from build123d import *

# Parameters (mm, degrees)
F0_R     = 2.013664
F1_DEPTH = 0.508
F2_R     = 2.54


with BuildPart() as f1:
    # F0 (on Top) → F1 (new body)
    with BuildSketch(Plane.XY):
        Polygon((5.08, 9.940335), (-3.64114, 9.940335), (-4.115906, 9.940335), (-4.115906, -0.219665), (5.08, -0.219665), align=None)
        with Locations((0, 5.06829)):
            Circle(F0_R, mode=Mode.SUBTRACT)
    extrude(amount=F1_DEPTH)

    # F2
    f2_edges = [f1.edges().sort_by_distance(p)[0] for p in [
        (5.08, 9.940335, 0.254),
        (5.08, -0.219665, 0.254),
    ]]
    fillet(f2_edges, radius=F2_R)


solid = f1.part
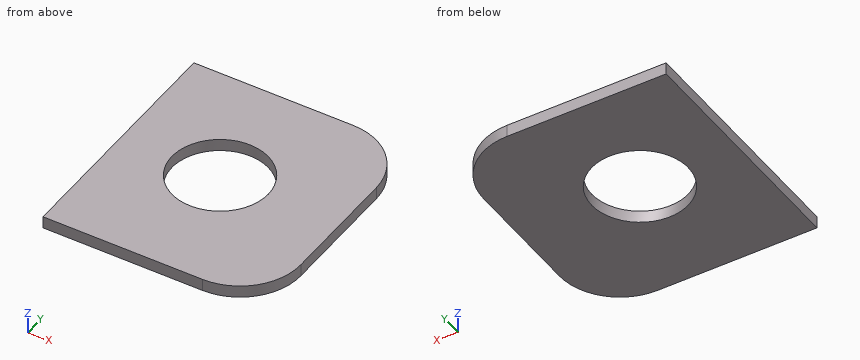
Design review of the part built by this model. Coordinates are the model's own, in mm. Round coordinates to 2 decimals unless told otherwise and drop trailing zeros. Write each loop counter-clockwise with the first axis right and the second up, starting at its lowest first coordinate (ties: lowest second). Pieces come first, ordered by that corner, then holes. Notation, with made-up numbers: (49.25, 43) - (92.25, 43) arc R19 cw to (92.25, 67) - close; hole circle Ø2 at (16.5, 88.25). An arc over 180 degrees is marked (long way). Use a Markdown table: item, result. Add a question column.
1. We need section D-D (y = 9.5). State the section outline as (x, z) points.
2. We need section A-A (x = 0). State the section outline as (y, z) points, then the cut area to 3 significant figures.
3. Wall thickness on probe 1 along Y at (x, z) = (0, 0.35); probe 2 along X at (y, z) = (5, 0.1); probe 3 along X at (y, z) = (3.75, 0.2): over which ranges is each line inside the solid? List them lowest first.
4. We need section C-C (z = 0.2). State the section outline as (x, y) points, then the cut area to 3 significant figures.
5. We need section B-B (y = 4.25). State the section outline as (x, z) points, then the cut area to 3 significant figures.
Output:
| question | item | result |
|---|---|---|
| 1 | outline | (-4.12, 0) - (3.97, 0) - (3.97, 0.51) - (-4.12, 0.51) - close |
| 2 | outline | (-0.22, 0) - (3.05, 0) - (3.05, 0.51) - (-0.22, 0.51) - close; (7.08, 0) - (9.94, 0) - (9.94, 0.51) - (7.08, 0.51) - close |
| 2 | area | 3.12 mm2 |
| 3 | probe 1 | y = -0.22 to 3.05, 7.08 to 9.94 |
| 3 | probe 2 | x = -4.12 to -2.01, 2.01 to 5.08 |
| 3 | probe 3 | x = -4.12 to -1.52, 1.52 to 5.08 |
| 4 | outline | (-4.12, -0.22) - (2.54, -0.22) arc R2.54 ccw to (5.08, 2.32) - (5.08, 7.4) arc R2.54 ccw to (2.54, 9.94) - (-4.12, 9.94) - close; hole circle Ø4.03 at (0, 5.07) |
| 4 | area | 77.9 mm2 |
| 5 | outline | (-4.12, 0) - (-1.84, 0) - (-1.84, 0.51) - (-4.12, 0.51) - close; (1.84, 0) - (5.08, 0) - (5.08, 0.51) - (1.84, 0.51) - close |
| 5 | area | 2.80 mm2 |
